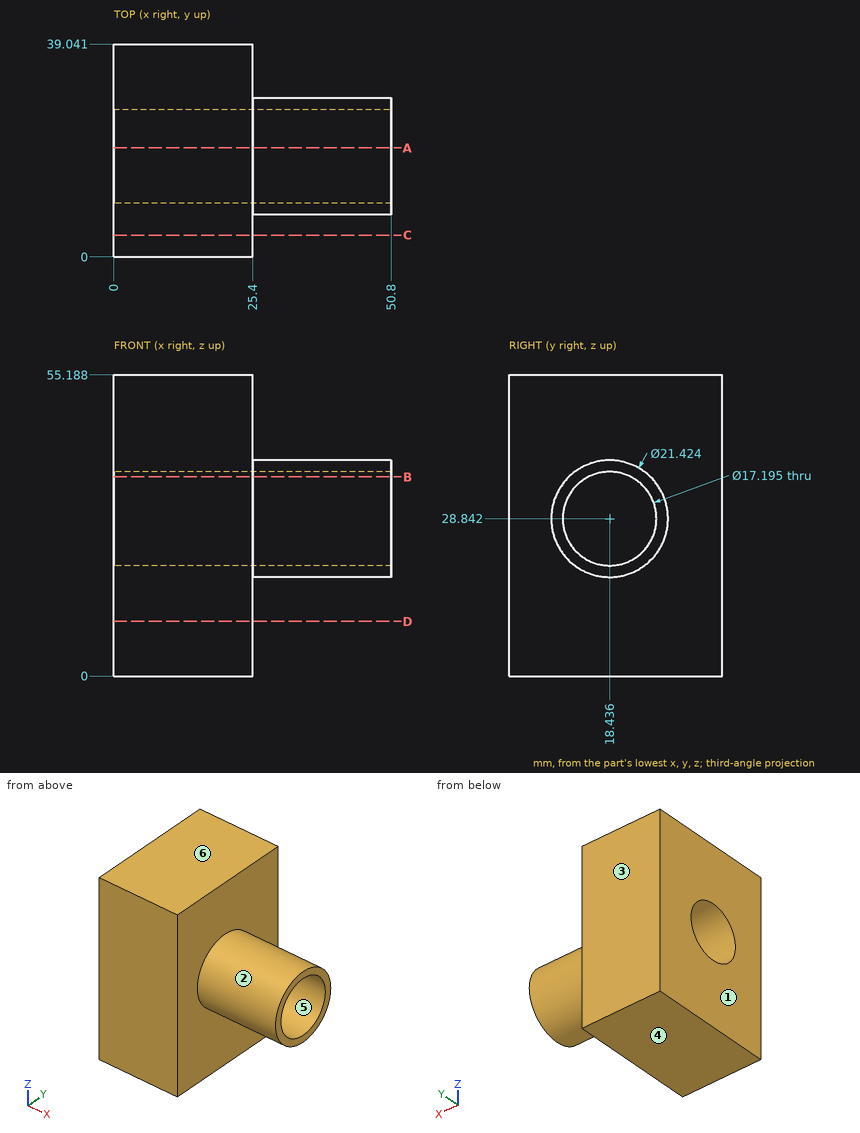
Study the drawing (mm; zero at the part's minimum x, y, z) and answer. A direction names the side the tool comes from. Give positions to 0.01 mm unless a question says otherwise; leave off trailing zeros. Write each loop counter-clockwise with the first axis right and the second up, starting at its lowest first coordinate (ties: lowest second). Pieces come first, ordered by that corner, then holes. Notation, with made-up numbers: M -39,15.5 L -5,15.5 A18 ccw -5,41.5 Z; hole C 14.5,16 d3. An arc over 180 degrees is marked long. Put each result on its own line as item: value. Start each with the question number.
1. The part is cut by section D-D, the plane z = 10. Give the vertices of the cut face in (x, y).
2. The part is cut by section B-B, the plane z = 36.5. Give the vertices of the cut face in (x, y) (1 decimal).
3. The part is cut by section A-A, the plane y = 20. Give the vertices of the cut face in (x, z) (1 decimal), and give its area (3 significant figures).
4. Each of these flat-tipped pins is pushed along its axis until it touches: pin 1 Ø6 at (x, z) = (15.5, 36) entering from -Y; pin 2 Ø10 at (x, z) = (36, 29) entering from -Y; pin 3 Ø12 at (x, y) = (35, 5) entering from -Z; pin 4 Ø4 at (x, y) = (35.5, 27.5) entering from +Z (1 decimal). Where does it stop, or does it pass through?
5. Consider line 1 along Z through (x, y) = (27.5, 18) (1 decimal); line 2 along X through (y, z) = (4.5, 22); line 3 along Z through (x, y) = (14, 24) (1 decimal). Determine where each line is inside the solid, lowest interval first.
6. The part is cut by section C-C, the plane y = 4. Give the vertices of the cut face in (x, z).
7. For a pull along Z with two mould halves and no side action, classify the marked faces 3, 4, 5 and 6 as released by +Z, released by -Z, zero draft, split by the parting line, or undercut.
8. Which of the six approach directions +Z, -Z, +X, -X, +Y, -Y give full straight-line access (tool end or side, diameter ignored) to the marked faces 1 and 2?
Final values:
1. outline: M 0,0 L 25.4,0 L 25.4,39.04 L 0,39.04 Z
2. outline: M 0,0 L 25.4,0 L 25.4,10.9 L 50.8,10.9 L 50.8,14.5 L 0,14.5 Z; M 0,22.3 L 50.8,22.3 L 50.8,25.9 L 25.4,25.9 L 25.4,39 L 0,39 Z
3. outline: M 0,0 L 25.4,0 L 25.4,18.2 L 50.8,18.2 L 50.8,20.4 L 0,20.4 Z; M 0,37.3 L 50.8,37.3 L 50.8,39.4 L 25.4,39.4 L 25.4,55.2 L 0,55.2 Z
3. area: 1,080 mm²
4. pin 1: stops at y = 0
4. pin 2: stops at y = 7.72
4. pin 3: stops at z = 21.13
4. pin 4: stops at z = 36.9
5. line 1: z = 18.1 to 20.3, 37.4 to 39.5
5. line 2: x = 0 to 25.4
5. line 3: z = 0 to 22.3, 35.4 to 55.2
6. outline: M 0,0 L 25.4,0 L 25.4,55.19 L 0,55.19 Z
7. face 3: zero draft
7. face 4: released by -Z
7. face 5: undercut
7. face 6: released by +Z
8. face 1: +Z, -Z, -X, +Y, -Y
8. face 2: +X
